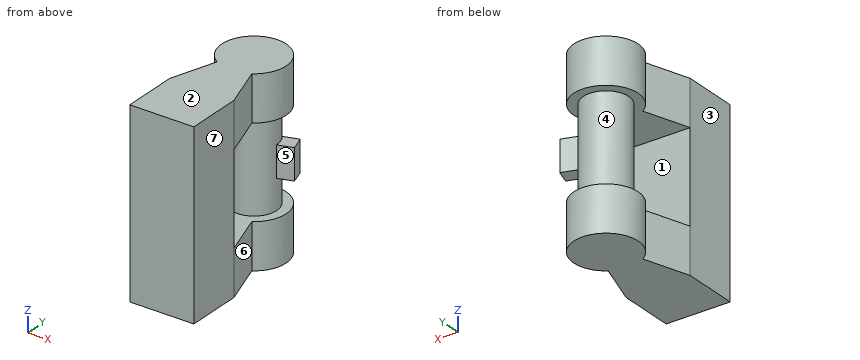
Autodesk Inventor part; units mm, degrees
ref_plane "YZ Plane" through (0, 0, 0) normal (1, 0, 0) x (0, 1, 0)
ref_plane "XZ Plane" through (0, 0, 0) normal (0, 1, 0) x (-1, 0, 0)
ref_plane "XY Plane" through (0, 0, 0) normal (0, 0, 1) x (1, 0, 0)
sketch "Sketch1" plane through (0, 0, 0) normal (0, 0, 1) x (1, 0, 0)
  line L0 (0, 0) -> (103.82, 0)
  line L1 (0, 0) -> (0, 89.86)
  line L2 (103.82, 89.86) -> (103.82, 0)
  line L3 (103.82, 89.86) -> (80.0424, 163.0401)
  line L4 (0, 89.86) -> (23.7776, 163.0401)
  line L5 (0, 89.86) -> (103.82, 89.86)
  arc A0 (80.0424, 163.0401) -> (23.7776, 163.0401) centre (51.91, 206.88) ccw
  dimension "d1" = 89.86
sketch "Sketch2" plane through (0, 0, 0) normal (0, 0, 1) x (1, 0, 0)
  circle A0 centre (51.91, 206.8113) radius 52.09
  line L0 (0, 89.8599) -> (24.0879, 163.9947)
  line L1 (0, 89.8599) -> (77.95, 89.8599) construction
  point P0 (0, 0)
extrude "Extrusion1" add sketch "Sketch1" along normal blind 294.64
sketch "Sketch3" plane through (103.82, 0, 0) normal (1, 0, 0) x (0, 0, -1)
  line L0 (-294.64, 89.86) -> (-294.64, 0)
  line L1 (0, 89.86) -> (-294.64, 89.86)
  line L2 (-220.98, 89.86) -> (-73.66, 89.86)
  line L3 (-73.66, 89.86) -> (-73.66, 276.7764)
  line L4 (-73.66, 276.7764) -> (-220.98, 276.7764)
  line L5 (0, 163.0401) -> (-294.64, 163.0401)
  line L6 (-220.98, 276.7764) -> (-220.98, 89.86)
  point P0 (0, 0)
extrude "Extrusion2" cut sketch "Sketch3" along normal mid plane 294.64
sketch "Sketch4" plane through (0, 0, 0) normal (0, 0, -1) x (-1, 0, 0)
  point P0 (0, 0)
sketch "Sketch5" plane through (0, 0, 0) normal (0, 0, -1) x (-1, 0, 0)
  point P0 (0, 0)
sketch "Sketch6" plane through (0, 0, 294.64) normal (0, 0, 1) x (1, 0, 0)
  point P0 (0, 0)
sketch "Sketch7" plane through (51.91, 206.88, 73.66) normal (0, 0, 1) x (1, 0, 0)
  circle A0 centre (0, 0) radius 36.83
  point P0 (-51.91, -206.88)
  dimension "d23" = 73.66
extrude "Extrusion3" cut sketch "Sketch7" against normal blind 30
sketch "Sketch8" plane through (51.91, 206.88, 220.98) normal (0, 0, -1) x (-1, 0, 0)
  circle A0 centre (0, 0) radius 36.83
  point P0 (51.91, -206.88)
  dimension "d26" = 73.66
extrude "Extrusion4" cut sketch "Sketch8" against normal blind 30
sketch "Sketch9" plane through (51.91, 206.88, 250.98) normal (0, 0, -1) x (-1, 0, 0)
  circle A0 centre (0, 0) radius 36.83
  point P0 (51.91, -206.88)
  dimension "d29" = 73.66
extrude "Extrusion5" add sketch "Sketch9" along normal blind 207.32
ref_plane "Work Plane2" through (86.148, 100.9846, 220.98) normal (0.9511, 0.309, 0) x (0, 0, -1)
ref_plane "Work Plane1" through (51.91, 89.86, 220.98) normal (0.9511, 0.309, 0) x (0, 0, -1)
sketch "Sketch10" plane through (86.148, 100.9846, 220.98) normal (0.9511, 0.309, 0) x (0, 0, -1)
  line L0 (0, 148.1226) -> (0, 74.4626) construction
  line L1 (0, 111.2926) -> (147.32, 111.2926) construction
  line L2 (147.32, 74.4626) -> (147.32, 148.1226) construction
  line L3 (0, 148.1226) -> (147.32, 148.1226) construction
  line L4 (73.66, 148.1226) -> (73.66, 74.4626) construction
  line L5 (0, 74.4626) -> (147.32, 74.4626) construction
  line L6 (73.66, 111.2926) -> (48.66, 111.2926) construction
  line L7 (48.66, 111.2926) -> (48.66, 123.5771) construction
  line L8 (48.66, 123.5771) -> (98.66, 123.5771)
  line L9 (98.66, 123.5771) -> (98.66, 99.0081)
  line L10 (98.66, 99.0081) -> (48.66, 99.0081)
  line L11 (48.66, 99.0081) -> (48.66, 123.5771)
  point P0 (220.98, -69.4209)
  dimension "d33" = 25
  dimension "d34" = 12.2845
  dimension "d35" = 50
  dimension "d36" = 24.569
extrude "Extrusion6" add sketch "Sketch10" along normal blind 60
properties part number "Dish antenna base"
Part model, mm, in its own coordinate system. Face numbers are marked on the shaded views. A direction names the side the tool comes from. Round coordinates to 2 decimals unless told otherwise and drop trailing zeros. Order: outer loops, then holes, each group sorted by start corner. A loop starts at its lowest first (then second) coordinate and runs counter-clockwise, first axis right, second up. Notation, with made-up numbers: M -30,-38 L 0,-38 A19 cw 0,-18 Z; hole C 66,-31.5 d11. An arc over 180 degrees is marked long. Put each result on its own line as item: value. Start each with the question number.
1. Slice it at C-C on y = 178.5. List the corners of the cut face in (x, z).
2. Tool access for the marked faces 5, 6 and 7: list every direction of +Z, -Z, +X, -X, +Y, -Y with a clear straight run to the whole face (end or side of a thin tool).
3. Slice it at A-A on x = 51.91. List the corners of the cut face in (y, z), then the cut area to 3 significant figures.
4. Slice it at B-B on z = 200. List the corners of the cut face in (x, y).
5. Slice it at D-D on z = 64. List the corners of the cut face in (x, y), then the cut area to 3 significant figures.
6. Drop flat-ended pins along their axis: pin 1 (2 mm diameter, centred on y = 133.5, z = 54.5, fed in from -X); pin 2 (8 mm diameter, centred on x = 95.5, z = 195.5, fed in from +Y). Give the stop position or say it passes through.
7. Drill centre lines: probe 1 along Z at (x, y) = (11, 105); probe 2 along Y at (x, z) = (71, 96.5); probe 3 along Y at (x, z) = (10, 162). Where is each one in solid material? Low to high. Write a range as [from, to].
8. Two-plate mould, pull along Z, no slides. Class the marked faces 1, 2, 3 and 4: +Z half, -Z half, draft (parallel to the pull), parting line (faces both ways), or undercut.
Findings:
1. outline: M 8.23,0 L 95.59,0 L 95.59,73.66 L 75.38,73.66 L 75.38,220.98 L 95.59,220.98 L 95.59,294.64 L 8.23,294.64 L 8.23,220.98 L 28.44,220.98 L 28.44,73.66 L 8.23,73.66 Z
2. face 5: +X
2. face 6: +Z, -Z, +X
2. face 7: +Z, -Z, +X, -Y
3. outline: M 0,0 L 258.97,0 L 258.97,73.66 L 243.71,73.66 L 243.71,220.98 L 258.97,220.98 L 258.97,294.64 L 0,294.64 Z; hole M 89.86,73.66 L 170.05,73.66 L 170.05,220.98 L 89.86,220.98 Z
3. area: 62,200 mm2
4. outline: M 0,0 L 103.82,0 L 103.82,89.86 L 0,89.86 Z; C 51.91,206.88 d73.66
5. outline: M 0,0 L 103.82,0 L 103.82,89.86 L 80.04,163.04 A52.09 ccw long 23.78,163.04 L 0,89.86 Z
5. area: 23,400 mm2
6. pin 1: x = 13.85
6. pin 2: y = 89.86
7. probe 1: [0, 73.66], [220.98, 294.64]
7. probe 2: [0, 89.86], [175.38, 238.38]
7. probe 3: [0, 89.86]
8. face 1: undercut
8. face 2: +Z half
8. face 3: draft
8. face 4: undercut
